Model file for the job. Use its own axes, mm. A direction names the side the tool comes from. Give positions to 0.01 mm unless a question says otherwise; leave off trailing zeros. Write each loop counter-clockwise with the first axis right and the second up, starting at its lowest first coordinate (ties: lowest second). Pieces come first, ordered by that corner, then holes.
```python
from build123d import *

# Parameters (mm, degrees)
SKETCH1_W             = 8
SKETCH1_H             = 8
SKETCH1_R             = 1.25
BOSS_EXTRUDE1_DEPTH   = 40
BOSS_EXTRUDE1_2_DEPTH = 40
BOSS_EXTRUDE2_DEPTH   = 8
SKETCH3_W             = 3.329640508
SKETCH3_H             = 8
BOSS_EXTRUDE3_DEPTH   = 8
SKETCH4_R             = 1.5
CUT_EXTRUDE1_DEPTH    = 6


with BuildPart() as part:
    # Sketch1 → Boss-Extrude1 (new body)
    with BuildSketch(Plane.XY):
        with Locations((0, 21)):
            Rectangle(SKETCH1_W, SKETCH1_H)
        with Locations((0, 21)):
            Circle(SKETCH1_R, mode=Mode.SUBTRACT)
    extrude(amount=BOSS_EXTRUDE1_DEPTH)



with BuildPart() as body_2:
    # Sketch1 → Boss-Extrude1 2 (new body)
    with BuildSketch(Plane.XY):
        with Locations((0, -21)):
            Rectangle(SKETCH1_W, SKETCH1_H)
        with Locations(Location((0, -21, 0), (0, 0, 180))):
            Circle(SKETCH1_R, mode=Mode.SUBTRACT)
    extrude(amount=BOSS_EXTRUDE1_2_DEPTH)


with BuildPart() as part_1:
    add(part.part)

    add(body_2.part)  # Boss-Extrude2 merges body 2
    # Sketch2 → Boss-Extrude2 (add)
    with BuildSketch(Plane.ZY.offset(4)):
        with BuildLine():
            Line((3.329640508, 17), (11.063985021, 17))
            ThreePointArc((11.063985021, 17), (14.56966913, 10.077818269), (16.196928044, 2.491089763))
            Line((16.196928044, 2.491089763), (23.803071956, 2.491089763))
            ThreePointArc((23.803071956, 2.491089763), (25.43033087, 10.077818269), (28.936014979, 17))
            Line((28.936014979, 17), (36.670359492, 17))
            ThreePointArc((36.670359492, 17), (29.700211914, 0), (36.670359492, -17))
            Line((36.670359492, -17), (28.936014979, -17))
            ThreePointArc((28.936014979, -17), (25.433314102, -10.086246784), (23.804551435, -2.508910237))
            Line((23.804551435, -2.508910237), (16.195448565, -2.508910237))
            ThreePointArc((16.195448565, -2.508910237), (14.566685898, -10.086246784), (11.063985021, -17))
            Line((11.063985021, -17), (3.329640508, -17))
            ThreePointArc((3.329640508, -17), (10.299788086, 0), (3.329640508, 17))
        make_face()
    extrude(amount=-BOSS_EXTRUDE2_DEPTH)

    # Sketch3 → Boss-Extrude3 (add)
    with BuildSketch(Plane(origin=(4, 0, 0), x_dir=(0, 0, -1), z_dir=(1, 0, 0))):
        with Locations((-38.335179746, 21)):
            Rectangle(SKETCH3_W, SKETCH3_H)
    extrude(amount=BOSS_EXTRUDE3_DEPTH)

    # Sketch4 → Cut-Extrude1 (cut)
    with BuildSketch(Plane(origin=(0, 0, 36.670359492), x_dir=(-1, 0, 0), z_dir=(0, 0, -1))):
        with Locations((-9, 21)):
            Circle(SKETCH4_R)
    extrude(amount=-CUT_EXTRUDE1_DEPTH, mode=Mode.SUBTRACT)


solid = part_1.part
```
1. Pin check, flat tips, straight feed: P1, Ø6, axis at x = 8.5, z = 33, coming from the -Y side; P2, Ø5, axis at x = 5.5, y = 2.5, coming from the -Z side; P3, Ø6.5, axis at x = 7.5, y = 21, coming from the -Z side; P4, Ø12, axis at y = 0.5, z = 26, coming from the +X side. Stop position of each tip, or through.
Calculated:
P1: passes through
P2: stops at z = 9.88
P3: stops at z = 36.67
P4: stops at x = 4
2. Which spindle directions (+Z, -Z, +X, -X, +Y, -Y) get a long thin tool onto all of the face, cutting with end or side? Do faces 4 (the flat face through (-1, -20, 0)), 5 (the flat face through (4, 21, 40)), 6 (the flat face through (7, 21, 36.67)), 7 (the flat face through (0, -17, 20)), 8 (the flat face through (0, -17, 38)). Say none if no direction does.
Calculated:
face 4: -Z, +X, -X, +Y, -Y
face 5: +Z, +X, -X, +Y, -Y
face 6: -Z, +X, +Y, -Y
face 7: +X, -X
face 8: +Z, +X, -X
3. Slice it at D-D, the plane z = 5.5. Write the cut outline in (x, y), and give its area (3 significant figures).
Calculated:
outline: (-4, -25) - (4, -25) - (4, -14.47) - (-4, -14.47) - close; (-4, 14.47) - (4, 14.47) - (4, 25) - (-4, 25) - close; hole circle Ø2.5 at (0, -21); hole circle Ø2.5 at (0, 21)
area: 159 mm2
4. Slice it at B-B, the plane y = -21. Write the cut outline in (x, z).
Calculated:
outline: (-4, 0) - (-1.25, 0) - (-1.25, 40) - (-4, 40) - close; (1.25, 0) - (4, 0) - (4, 40) - (1.25, 40) - close
5. Probe probe 1 along Y at (x, z) = (2.25, 19.5); probe 2 along Y at (x, z) = (0, 29); probe 3 along Y at (x, z) = (9, 37.8). List the from-to ranges inside material, lowest first.
Calculated:
probe 1: y = -25 to -17, -2.51 to 2.49, 17 to 25
probe 2: y = -25 to -22.25, -19.75 to 19.75, 22.25 to 25
probe 3: y = 17 to 19.5, 22.5 to 25
6. Slice it at A-A, the plane x = 0. Write the cut outline in (y, z), and give its area (3 significant figures).
Calculated:
outline: (-25, 0) - (-22.25, 0) - (-22.25, 40) - (-25, 40) - close; (-19.75, 0) - (-17, 0) - (-17, 3.33) arc R24.22 cw to (17, 3.33) - (17, 0) - (19.75, 0) - (19.75, 40) - (17, 40) - (17, 36.67) arc R24.22 cw to (-17, 36.67) - (-17, 40) - (-19.75, 40) - close; (22.25, 0) - (25, 0) - (25, 40) - (22.25, 40) - close; hole (-17, 11.06) arc R30.22 cw to (-2.51, 16.2) - (-2.51, 23.8) arc R30.22 cw to (-17, 28.94) - close; hole (2.49, 16.2) arc R30.22 cw to (17, 11.06) - (17, 28.94) arc R30.22 cw to (2.49, 23.8) - close
area: 919 mm2
7. Slice it at C-C, the plane z = 20. Write the cut outline in (x, y), and give its area (3 significant figures).
Calculated:
outline: (-4, -25) - (4, -25) - (4, -17) - (-4, -17) - close; (-4, -2.51) - (4, -2.51) - (4, 2.49) - (-4, 2.49) - close; (-4, 17) - (4, 17) - (4, 25) - (-4, 25) - close; hole circle Ø2.5 at (0, -21); hole circle Ø2.5 at (0, 21)
area: 158 mm2
8. Pull direction X, two halves, no side cores. Call faces 1 (the cylindrical face through (-0.27, 19.78, 19.72)), 2 (the flat face through (-4, 0, 20)), 3 (the flat face through (0, 2.491, 20)): +X half, -X half, draft (parallel to the pull), parting line (faces both ways), or undercut.
Calculated:
face 1: undercut
face 2: -X half
face 3: draft
